```python
from build123d import *

# Parameters (mm, degrees)
SKETCH1_R           = 26.5
BOSS_EXTRUDE1_DEPTH = 56
SKETCH4_R           = 37.5
BOSS_EXTRUDE2_DEPTH = 5
SKETCH5_R           = 8.5
CUT_EXTRUDE1_DEPTH  = 81.830068663
CUT_EXTRUDE2_DEPTH  = 5


with BuildPart() as part:
    # Sketch1 → Boss-Extrude1 (new body)
    with BuildSketch(Plane.XY):
        Circle(SKETCH1_R)
    extrude(amount=BOSS_EXTRUDE1_DEPTH)

    # Sketch4 → Boss-Extrude2 (add)
    with BuildSketch(Plane(origin=(0, 0, 0), x_dir=(-1, 0, 0), z_dir=(0, 0, -1))):
        Circle(SKETCH4_R)
    extrude(amount=BOSS_EXTRUDE2_DEPTH)

    # Sketch5 → Cut-Extrude1 (cut, through all)
    with BuildSketch(Plane.XY.offset(56)):
        Circle(SKETCH5_R)
    extrude(amount=-CUT_EXTRUDE1_DEPTH, mode=Mode.SUBTRACT)

    # Sketch6 → Cut-Extrude2 (cut, symmetric)
    with BuildSketch(Plane(origin=(0, 0, 0), x_dir=(1, 0, 0), z_dir=(0, 1, 0))):
        Polygon((23.5, -56), (26.5, -56), (26.5, -36), (21.5, -36), (21.5, -39.5), (23.5, -41.5), align=None)
    cut_extrude2 = extrude(amount=CUT_EXTRUDE2_DEPTH, both=True, mode=Mode.SUBTRACT)

    # Mirror1: Cut-Extrude2 across plane
    add(cut_extrude2.mirror(Plane(origin=(0, 0, 0), x_dir=(0, 0, 1), z_dir=(1, 0, 0))), mode=Mode.SUBTRACT)


solid = part.part
```
The model under review builds one solid part; all positions refer to its coordinate system, in mm. A direction names the side the tool comes from. Round coordinates to 2 decimals unless told otherwise and drop trailing zeros. Loops run counter-clockwise (first coordinate to the right, second up) from the corner with the lowest first, then second, coordinate; pieces in that order, holes last. Notation, with made-up numbers: M 54.5,-11 L 93.5,-11 A22 cw 93.5,17 Z; hole C 58.25,-3 d9. An arc over 180 degrees is marked long. Put each result on its own line as item: value.
Q1. Consider section A-A, the plane y = 0. Give the boundary of the cut face in (x, z).
Result set:
outline: M -37.5,-5 L -8.5,-5 L -8.5,56 L -23.5,56 L -23.5,41.5 L -21.5,39.5 L -21.5,36 L -26.5,36 L -26.5,0 L -37.5,0 Z; M 8.5,-5 L 37.5,-5 L 37.5,0 L 26.5,0 L 26.5,36 L 21.5,36 L 21.5,39.5 L 23.5,41.5 L 23.5,56 L 8.5,56 Z
Q2. Consider section D-D, the plane y = 10. Give the boundary of the cut face in (x, z), then the cut area to 3 significant figures.
Result set:
outline: M -36.14,-5 L 36.14,-5 L 36.14,0 L 24.54,0 L 24.54,56 L -24.54,56 L -24.54,0 L -36.14,0 Z
area: 3,110 mm²
Q3. To check wall thickness, follow L1, parallel to Y at x = 0, z = 22; L2, parallel to Z at x = -17, y = -27; L3, parallel to Y at x = 7, z = 18. State the ranges of each line that lie inside material, in increasing order.
Result set:
L1: y = -26.5 to -8.5, 8.5 to 26.5
L2: z = -5 to 0
L3: y = -25.56 to -4.82, 4.82 to 25.56
Q4. Machinability: for faces 1 (the flat face through (-23.5, 0, 49)), 2 (the flat face through (-24, -5, 44)), 3 (the flat face through (21.5, 0, 38)), 4 (the flat face through (23.5, 0, 49)), which of the approach directions +Z, -Z, +X, -X, +Y, -Y give a long, thin tool a straight path to every point of the face, cutting with its end or side? Answer none if there is none.
Result set:
face 1: +Z, -X
face 2: -X
face 3: +X
face 4: +Z, +X
Q5. Consider section C-C, the plane z = 10.5. Give the boundary of the cut face in (x, y), then the cut area to 3 significant figures.
Result set:
outline: C 0,0 d53; hole C 0,0 d17
area: 1,980 mm²
Q6. Mouldability with a two-part tool opening along Y and no side actions: class faces 5 (the flat face through (-8, 26, 0)), 6 (the flat face through (24, 0, 36)), 7 (the cylindrical face through (25.276, 7.96, 27.608)), 8 (the flat face through (-21.5, 0, 38)) as released by +Y, released by -Y, zero draft, split by the parting line, or undercut.
Result set:
face 5: zero draft
face 6: undercut
face 7: split by the parting line
face 8: undercut
Q7. For pin 1 (6 mm diameter, centred on y = 25, z = 32, fed in from +X); pin 2 (3.5 mm diameter, centred on x = 22.5, z = 49.5, fed in from +Y); pin 3 (2 mm diameter, centred on y = -20, z = 30, fed in from +X); pin 4 (15.5 mm diameter, centred on x = 0, y = 0, fed in from -Z), all flat-tipped, find the tip position at first contact; note any pin that passes through.
Result set:
pin 1: stops at x = 14.77
pin 2: stops at y = 16.48
pin 3: stops at x = 18.47
pin 4: passes through
Q8. Consider section B-B, the plane x = 0. Give the boundary of the cut face in (y, z), then the cut area to 3 significant figures.
Result set:
outline: M -37.5,-5 L -8.5,-5 L -8.5,56 L -26.5,56 L -26.5,0 L -37.5,0 Z; M 8.5,-5 L 37.5,-5 L 37.5,0 L 26.5,0 L 26.5,56 L 8.5,56 Z
area: 2,310 mm²
